Source: CAD feature listing. Evaluate the final solid. Frame: model axes, mm. A direction names the side the tool comes from. Round coordinates to 2 decimals unless told otherwise and drop trailing zeros. Write each loop counter-clockwise with the first axis right and the second up, starting at its lowest first coordinate (ties: lowest second). Pieces come first, ordered by that corner, then holes.
from build123d import *

# Parameters (mm, degrees)
SKETCH1_R           = 25
BOSS_EXTRUDE1_DEPTH = 40
CUT_EXTRUDE1_START  = -8.7
SKETCH2_R           = 25
SKETCH2_R_2         = 4.85
CUT_EXTRUDE1_DEPTH  = 8.7
CUT_EXTRUDE2_DEPTH  = 10
SKETCH5_R           = 1.5
CUT_EXTRUDE3_DEPTH  = 42.275779823


with BuildPart() as part:
    # Sketch1 → Boss-Extrude1 (new body)
    with BuildSketch(Plane(origin=(0, 0, 0), x_dir=(1, 0, 0), z_dir=(0, 1, 0))):
        with Locations(Location((0, 0, 0), (0, 0, 270))):
            Circle(SKETCH1_R)
    extrude(amount=BOSS_EXTRUDE1_DEPTH)

    # Sketch2 → Cut-Extrude1 (cut)
    with BuildSketch(Plane(origin=(0, 40, 0), x_dir=(1, 0, 0), z_dir=(0, 1, 0)).offset(CUT_EXTRUDE1_START)):
        with Locations(Location((0, 0, 0), (0, 0, 270))):
            Circle(SKETCH2_R)
        with Locations(Location((0, 0, 0), (0, 0, 270))):
            Circle(SKETCH2_R_2, mode=Mode.SUBTRACT)
    extrude(amount=CUT_EXTRUDE1_DEPTH, mode=Mode.SUBTRACT)

    # Sketch3 → Cut-Extrude2 (cut)
    with BuildSketch(Plane(origin=(0, 31.3, 0), x_dir=(1, 0, 0), z_dir=(0, 1, 0))):
        with BuildLine():
            Line((-2.6, -15), (-2.6, -20))
            ThreePointArc((-2.6, -20), (0, -22.6), (2.6, -20))
            Line((2.6, -20), (2.6, -15))
            ThreePointArc((2.6, -15), (0, -12.4), (-2.6, -15))
        make_face()
    extrude(amount=-CUT_EXTRUDE2_DEPTH, mode=Mode.SUBTRACT)

    # Sketch5 → Cut-Extrude3 (cut, through all)
    with BuildSketch(Plane(origin=(0, 21.3, 0), x_dir=(1, 0, 0), z_dir=(0, 1, 0))):
        with Locations(Location((0, -17.5, 0), (0, 0, 270))):
            Circle(SKETCH5_R)
    extrude(amount=-CUT_EXTRUDE3_DEPTH, mode=Mode.SUBTRACT)


solid = part.part
1) Material intervals for line 1 (Y direction, x = -7.5, z = 21.5); line 2 (X direction, y = 7.5, z = 17.5); line 3 (X direction, y = 31, z = 18.5), sorted ascending.
Taken from the geometry:
line 1: y = 0 to 31.3
line 2: x = -17.85 to -1.5, 1.5 to 17.85
line 3: x = -16.82 to -2.6, 2.6 to 16.82
2) Section query C-C on y = 5.5. Return the cut outline in (x, z), then the cut area to 3 significant figures.
Taken from the geometry:
outline: circle Ø50 at (0, 0); hole circle Ø3 at (0, 17.5)
area: 1,960 mm2
3) Contact query for flat-ended pins moving along their axis: P1, Ø1.6, axis at x = 1, z = 18.5, coming from the +Y side; P2, Ø10, axis at y = 17.5, z = 8, coming from the -X side; P3, Ø4, axis at y = 28.5, z = 17.5, coming from the +X side. Output: stop coordinate, or through.
Taken from the geometry:
P1: stops at y = 21.3
P2: stops at x = -24.82
P3: stops at x = 19.62
4) Section query D-D on x = -15. Return the cut outline in (y, z).
Taken from the geometry:
outline: (0, -20) - (31.3, -20) - (31.3, 20) - (0, 20) - close
5) Section query A-A on z = 18. Return the cut outline in (x, y).
Taken from the geometry:
outline: (-17.35, 0) - (-1.41, 0) - (-1.41, 21.3) - (-2.6, 21.3) - (-2.6, 31.3) - (-17.35, 31.3) - close; (1.41, 0) - (17.35, 0) - (17.35, 31.3) - (2.6, 31.3) - (2.6, 21.3) - (1.41, 21.3) - close
6) Pull-direction query (X, two-part tool) for faces 1 (the face through (-2.6, 26, 17)), 2 (the face through (0, 0, 0)), 3 (the face through (-0.1, 26.4, 22.6)), 4 (the face through (1.457, 35.589, 4.626)); classes: released by +X, released by -X, zero draft, split by the parting line, or undercut.
Taken from the geometry:
face 1: undercut
face 2: zero draft
face 3: undercut
face 4: split by the parting line
7) Reachability of faces 5 (the face through (2.6, 26, 18)), 6 (the face through (0, 40, 0)) from +Z, -Z, +X, -X, +Y, -Y: full face, straight path, thin tool, end or side. Return the list, or none.
Taken from the geometry:
face 5: +Y
face 6: +Z, -Z, +X, -X, +Y
8) Section query B-B on z = 0. Return the cut outline in (x, y).
Taken from the geometry:
outline: (-25, 0) - (25, 0) - (25, 31.3) - (4.85, 31.3) - (4.85, 40) - (-4.85, 40) - (-4.85, 31.3) - (-25, 31.3) - close
